Can you work these out from the model? Positions are in its coordinate system, mm. A direction names the side the tool comes from. Give positions to 0.01 mm unless a question says otherwise; leave off trailing zeros. Write each loop counter-clockwise with the first axis right and the second up, starting at its lowest first coordinate (ties: lowest second). Pieces come first, ordered by that corner, then holes. Notation, with made-up numbers: (-37, 69) -> (-6, 69) arc R5 cw to (-6, 76) -> close; hole circle Ø3 at (31.5, 59.5). An arc over 180 degrees is marked (long way). Answer as CSV lines item,"result". Start each with the question number.
1. On a 3-axis mill with a long thin cutter (end or side, diameter ignored), from which of +Z, -Z, +X, -X, +Y, -Y can I reach the whole of each face in a straight line? I mean faces 1 (the face through (0, 0, 40)), 2 (the face through (0, 0, 20)). Say none if no direction works.
2. If we section it at C-C on x = -0.75: Write out the boundary of the cut face in (y, z), plus the area to 3 significant figures.
3. I need wall thicknesses on line 1 (Y direction, x = 0, z = 6.5); line 2 (Z direction, x = 3.75, y = -1); line 3 (Z direction, x = 2.5, y = 5.25). Which ranges of each line are inside material? Lowest first, please. Write a range as [from, to].
4. If we mould it in two halves opening along Y, with no side actions, what happens to faces 3 (the face through (1.08, -4.88, 9.86)), 4 (the face through (3, 0, 22)), 5 (the face through (-0.454, -2.045, 30.874))? For each: pulls with the +Y half, pulls with the -Y half, needs draft (parallel to the pull), parting line crosses it, or undercut.
5. If we section it at D-D on z = 33.5: Write out the boundary of the cut face in (x, y) (3 decimals), plus the area to 3 significant figures.
6. I'm going to push flat-ended pins straight in: P1, Ø2, axis at x = -3.5, z = 19.5, coming from the -Y side; P2, Ø2, axis at y = -3.5, z = 13, coming from the -X side; P3, Ø3, axis at x = -2, y = -5, coming from the +Z side. Where does each tip first touch, or does it pass through?
7. If we section it at B-B on y = 0: Write out the boundary of the cut face in (x, z) (3 decimals), plus the area to 3 significant figures.
8. If we section it at A-A on z = 15.5: Write out the boundary of the cut face in (x, y), plus the area to 3 significant figures.
```python
from build123d import *

# Parameters (mm, degrees)
SKETCH5_R           = 6
BOSS_EXTRUDE4_DEPTH = 40
SKETCH6_R           = 5
CUT_EXTRUDE1_DEPTH  = 20
CUT_EXTRUDE2_START  = -18
SKETCH7_R           = 6
CUT_EXTRUDE2_DEPTH  = 18
SKETCH8_R           = 2.095
BOSS_EXTRUDE5_DEPTH = 18


with BuildPart() as part:
    # Sketch5 → Boss-Extrude4 (new body)
    with BuildSketch(Plane.XY):
        Circle(SKETCH5_R)
    extrude(amount=BOSS_EXTRUDE4_DEPTH)

    # Sketch6 → Cut-Extrude1 (cut)
    with BuildSketch(Plane(origin=(0, 0, 0), x_dir=(-1, 0, 0), z_dir=(0, 0, -1))):
        Circle(SKETCH6_R)
    extrude(amount=-CUT_EXTRUDE1_DEPTH, mode=Mode.SUBTRACT)

    # Sketch7 → Cut-Extrude2 (cut)
    with BuildSketch(Plane.XY.offset(40).offset(CUT_EXTRUDE2_START)):
        Circle(SKETCH7_R)
    extrude(amount=CUT_EXTRUDE2_DEPTH, mode=Mode.SUBTRACT)

    # Sketch8 → Boss-Extrude5 (add)
    with BuildSketch(Plane.XY.offset(22)):
        Circle(SKETCH8_R)
    extrude(amount=BOSS_EXTRUDE5_DEPTH)


solid = part.part
```
Computed values:
1,face 1,"+Z, +X, -X, +Y, -Y"
1,face 2,"-Z"
2,outline,"(-5.95, 0) -> (-4.94, 0) -> (-4.94, 20) -> (4.94, 20) -> (4.94, 0) -> (5.95, 0) -> (5.95, 22) -> (1.96, 22) -> (1.96, 40) -> (-1.96, 40) -> (-1.96, 22) -> (-5.95, 22) -> close"
2,area,"135 mm2"
3,line 1,"y = [-6, -5], [5, 6]"
3,line 2,"z = [20, 22]"
3,line 3,"z = [0, 22]"
4,face 3,"undercut"
4,face 4,"needs draft"
4,face 5,"parting line crosses it"
5,outline,"circle Ø4.19 at (0, 0)"
5,area,"13.8 mm2"
6,P1,"stops at y = -5.45"
6,P2,"stops at x = -5.45"
6,P3,"stops at z = 22"
7,outline,"(-6, 0) -> (-5, 0) -> (-5, 20) -> (5, 20) -> (5, 0) -> (6, 0) -> (6, 22) -> (2.095, 22) -> (2.095, 40) -> (-2.095, 40) -> (-2.095, 22) -> (-6, 22) -> close"
7,area,"139 mm2"
8,outline,"circle Ø12 at (0, 0); hole circle Ø10 at (0, 0)"
8,area,"34.6 mm2"
